Here's how the part is built. I have some questions about the finished solid (model axes, mm). A direction names the side the tool comes from. Round coordinates to 2 decimals unless told otherwise and drop trailing zeros. Order: outer loops, then holes, each group sorted by start corner. A loop starts at its lowest first (then second) coordinate and runs counter-clockwise, first axis right, second up.
```python
from build123d import *

# Parameters (mm, degrees)
SKETCH1_R                = 1.5
SKETCH1_R_2              = 12.5
BOSS_EXTRUDE1_DEPTH      = 4
SKETCH2_W                = 50
SKETCH2_H                = 25
SKETCH2_R                = 2
BOSS_EXTRUDE2_DEPTH      = 5
BOSS_EXTRUDE3_DEPTH      = 2
BOSS_EXTRUDE3_DEPTH_BACK = 2
SKETCH6_W                = 42
SKETCH6_H                = 42
CUT_EXTRUDE1_DEPTH       = 52.633322574
SKETCH6_3_W              = 20
SKETCH6_3_H              = 4
BOSS_EXTRUDE4_DEPTH      = 21


with BuildPart() as part:
    # Sketch1 → Boss-Extrude1 (new body)
    with BuildSketch(Plane.XY):
        Polygon((19.247712685, -19.276828776), (19.247712685, 19.723171224), (-19.752287315, 19.723171224), (-19.752287315, -19.276828776), (-10, -19.276828776), (-10, -40), (10, -40), (10, -19.276828776), align=None)
        with Locations((-15.752287315, 15.723171224)):
            Circle(SKETCH1_R, mode=Mode.SUBTRACT)
        with Locations((-15.752287315, -15.276828776)):
            Circle(SKETCH1_R, mode=Mode.SUBTRACT)
        with Locations((-0.252287315, 0.223171224)):
            Circle(SKETCH1_R_2, mode=Mode.SUBTRACT)
        with Locations((15.247712685, -15.276828776)):
            Circle(SKETCH1_R, mode=Mode.SUBTRACT)
        with Locations((15.247712685, 15.723171224)):
            Circle(SKETCH1_R, mode=Mode.SUBTRACT)
    extrude(amount=BOSS_EXTRUDE1_DEPTH)

    # Sketch2 → Boss-Extrude2 (add)
    with BuildSketch(Plane.XZ.offset(40)):
        with Locations((0, -8.5)):
            Rectangle(SKETCH2_W, SKETCH2_H)
        with Locations((-15, -14)):
            Circle(SKETCH2_R, mode=Mode.SUBTRACT)
        with Locations((15, -14)):
            Circle(SKETCH2_R, mode=Mode.SUBTRACT)
    extrude(amount=-BOSS_EXTRUDE2_DEPTH)

    # Sketch5 → Boss-Extrude3 (add, two sides: drawn at the far end of the back side and taken through both)
    with BuildSketch(Plane(origin=(0, 0, 0), x_dir=(0, 0, -1), z_dir=(1, 0, 0)).offset(-BOSS_EXTRUDE3_DEPTH_BACK)):
        Polygon((21, -35), (0, -12.250562953), (0, -35), align=None)
    extrude(amount=BOSS_EXTRUDE3_DEPTH + BOSS_EXTRUDE3_DEPTH_BACK)

    # Sketch6 → Cut-Extrude1 (cut, through all)
    with BuildSketch(Plane(origin=(0, 0, 0), x_dir=(-1, 0, 0), z_dir=(0, 0, -1))):
        Rectangle(SKETCH6_W, SKETCH6_H)
    extrude(amount=CUT_EXTRUDE1_DEPTH, mode=Mode.SUBTRACT)

    # Sketch6<3> → Boss-Extrude4 (add, through all)
    with BuildSketch(Plane(origin=(0, 0, 0), x_dir=(-1, 0, 0), z_dir=(0, 0, -1))):
        with Locations((0, -23)):
            Rectangle(SKETCH6_3_W, SKETCH6_3_H)
    extrude(amount=BOSS_EXTRUDE4_DEPTH)


solid = part.part
```
1. If we section it at C-C, the plane z = -15: Write out the boundary of the cut face in (x, y), and give its area (3 significant figures).
Evaluation:
outline: (-25, -40) - (-16.73, -40) - (-16.73, -35) - (-25, -35) - close; (-13.27, -40) - (13.27, -40) - (13.27, -35) - (2, -35) - (2, -28.5) - (-2, -28.5) - (-2, -35) - (-13.27, -35) - close; (-10, -25) - (10, -25) - (10, -21) - (-10, -21) - close; (16.73, -40) - (25, -40) - (25, -35) - (16.73, -35) - close
area: 321 mm2
2. If we section it at A-A, the plane x = 18: Write out the boundary of the cut face in (y, z), and give its area (3 significant figures).
Evaluation:
outline: (-40, -21) - (-35, -21) - (-35, 4) - (-40, 4) - close; (-19.28, 0) - (19.72, 0) - (19.72, 4) - (-19.28, 4) - close
area: 281 mm2
3. If we section it at B-B, the plane y = 4: Write out the boundary of the cut face in (x, z), and give its area (3 significant figures).
Evaluation:
outline: (-19.75, 0) - (-12.17, 0) - (-12.17, 4) - (-19.75, 4) - close; (11.66, 0) - (19.25, 0) - (19.25, 4) - (11.66, 4) - close
area: 60.7 mm2
4. If we mould it in two halves opening along Y, with no side actions, what happens to faces 1 (the cylindrical face through (16.68, 16.17, 1.97)), 2 (the flat face through (0, -21, -10)), 3 (the flat face through (-25, -38, -9))? For each: released by +Y, released by -Y, zero draft, split by the parting line, or undercut.
Evaluation:
face 1: undercut
face 2: released by +Y
face 3: zero draft
5. I'm going to push flat-ended pins straight in: P1, Ø3.5, axis at x = 15.25, y = 15.72, coming from the -Z side; P2, Ø1, axis at y = -26, z = -7, coming from the -X side; P3, Ø1.5, axis at x = 15, z = -12.5, coming from the +Y side; P4, Ø10, axis at x = 14, y = -27, coming from the -Z side. Where does each tip first touch, or does it pass through?
Evaluation:
P1: stops at z = 0
P2: stops at x = -2
P3: stops at y = -35
P4: stops at z = -21
6. On a 3-axis mill with a long thin cutter (end or side, diameter ignored), from which of +Z, -Z, +X, -X, +Y, -Y can I reach the whole of each face in a straight line? I mean faces 4 (the flat face through (-15, -19.277, 2)), 5 (the flat face through (6, -30, 0)), 6 (the flat face through (-2, -30, -8)), 7 (the flat face through (8.1, -9.4, 0)). Say none if no direction works.
Evaluation:
face 4: +Z, -Z, -X
face 5: -Z, +X
face 6: -Z, -X
face 7: -Z, +X, -X, +Y
7. I need wall thicknesses on probe 1 along Z at (x, y) = (-15, -36.1); probe 2 along Y at (x, z) = (-13, 2); probe 3 along Y at (x, z) = (-8.5, -17). Which ranges of each line are inside material? Lowest first, please.
Evaluation:
probe 1: z = -21 to -16, -12 to 4
probe 2: y = -40 to -35, -19.28 to 19.72
probe 3: y = -40 to -35, -25 to -21
8. If we section it at D-D, the plane z = -18: Write out the boundary of the cut face in (x, y).
Evaluation:
outline: (-25, -40) - (25, -40) - (25, -35) - (2, -35) - (2, -31.75) - (-2, -31.75) - (-2, -35) - (-25, -35) - close; (-10, -25) - (10, -25) - (10, -21) - (-10, -21) - close
